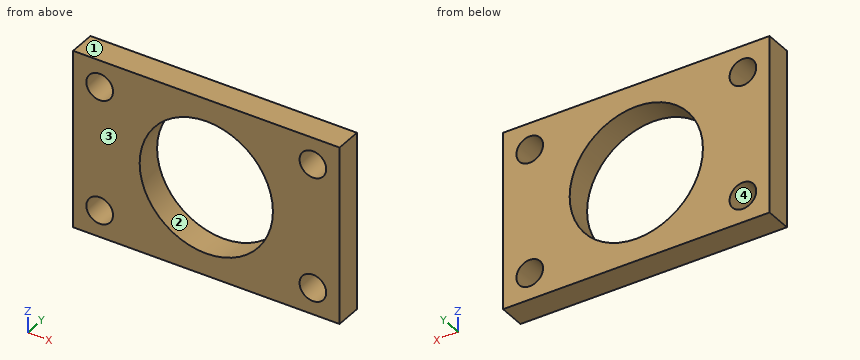
```python
from build123d import *

# Parameters (mm, degrees)
SKETCH1_W               = 30
SKETCH1_H               = 20
BOSS_EXTRUDE1_DEPTH     = 3
SKETCH2_R               = 1.5
SKETCH2_R_2             = 7.5
CUT_EXTRUDE1_DEPTH      = 3
CUT_EXTRUDE1_DEPTH_BACK = 23


with BuildPart() as part:
    # Sketch1 → Boss-Extrude1 (new body)
    with BuildSketch(Plane(origin=(0, 0, 0), x_dir=(1, 0, 0), z_dir=(0, 1, 0))):
        with Locations((-15, 10)):
            Rectangle(SKETCH1_W, SKETCH1_H)
    extrude(amount=BOSS_EXTRUDE1_DEPTH)

    # Sketch2 → Cut-Extrude1 (cut, two sides)
    with BuildSketch(Plane(origin=(0, 3, 0), x_dir=(1, 0, 0), z_dir=(0, 1, 0))) as cut_extrude1_sk:
        with Locations((-27, 17)):
            Circle(SKETCH2_R)
        with Locations((-27, 3)):
            Circle(SKETCH2_R)
        with Locations((-3, 3)):
            Circle(SKETCH2_R)
        with Locations((-3, 17)):
            Circle(SKETCH2_R)
        with Locations((-15, 10)):
            Circle(SKETCH2_R_2)
    extrude(amount=CUT_EXTRUDE1_DEPTH, mode=Mode.SUBTRACT)
    extrude(cut_extrude1_sk.sketch, amount=-CUT_EXTRUDE1_DEPTH_BACK, mode=Mode.SUBTRACT)


solid = part.part
```
Input: part model. Units: mm. Frame: model coordinates. Face numbers are marked on the shaded views. Coordinates: 2 decimals unless noted, no trailing zeros. Write each loop counter-clockwise with the first axis right and the second up, starting at its lowest first coordinate (ties: lowest second). Pieces come first, ordered by that corner, then holes. Notation, with made-up numbers: M 70,28 L 83,28 A26 ccw 83,65 Z; hole C 43,-35 d8. An arc over 180 degrees is marked long. Use one line per item in the form item = value.
Q1. First-contact query: pin 1 (1 mm diameter, centred on y = 2.5, z = -17, fed in from +X). Flat tip, straight axial feed; report the tip coordinate or a pass-through.
Answer below:
pin_1 = 0
Q2. Material intervals for probe 1 along Z at (x, y) = (-27, 1.4); probe 2 along X at (y, z) = (0.2, -16); probe 3 along Z at (x, y) = (-15, 2.1), sorted ascending. Write a range as from..to.
Answer below:
probe_1 = -20..-18.5, -15.5..-4.5, -1.5..0
probe_2 = -30..-28.12, -25.88..-19.5, -10.5..-4.12, -1.88..0
probe_3 = -20..-17.5, -2.5..0
Q3. Section B-B (z = -14.5). Return loops of the section in (x, y), plus the area to 3 significant figures.
Answer below:
outline = M -30,0 L -21,0 L -21,3 L -30,3 Z; M -9,0 L 0,0 L 0,3 L -9,3 Z
area = 54.0 mm²
Q4. Section D-D (x = -15). Return loops of the section in (y, z), plus the area to 3 significant figures.
Answer below:
outline = M 0,-20 L 3,-20 L 3,-17.5 L 0,-17.5 Z; M 0,-2.5 L 3,-2.5 L 3,0 L 0,0 Z
area = 15.0 mm²
Q5. Section C-C (y = 1.85). Return loops of the section in (x, z).
Answer below:
outline = M -30,-20 L 0,-20 L 0,0 L -30,0 Z; hole C -27,-17 d3; hole C -27,-3 d3; hole C -15,-10 d15; hole C -3,-17 d3; hole C -3,-3 d3
Q6. Draft query along Z for the marked faces 1, 2, 3 and 4. Return one class per face: released by +Z, released by -Z, zero draft, split by the parting line, or undercut.
Answer below:
face_1 = released by +Z
face_2 = undercut
face_3 = zero draft
face_4 = undercut
Q7. Section A-A (x = -3). Return loops of the section in (y, z), plus the area to 3 significant figures.
Answer below:
outline = M 0,-20 L 3,-20 L 3,-18.5 L 0,-18.5 Z; M 0,-15.5 L 3,-15.5 L 3,-4.5 L 0,-4.5 Z; M 0,-1.5 L 3,-1.5 L 3,0 L 0,0 Z
area = 42.0 mm²
